CAD build for the part. Positions are in the model's coordinates, mm. Round coordinates to 2 decimals unless told otherwise and drop trailing zeros. Loops run counter-clockwise (first coordinate to the right, second up) from the corner with the lowest first, then second, coordinate; pieces in that order, holes last. Notation, with made-up numbers: (80.5, 83) - (120.5, 83) arc R14 ccw to (120.5, 96) - close; hole circle Ø6 at (-13, 14). An arc over 180 degrees is marked (long way). Use one line per item in the form item = value.
Autodesk Fusion 360 part; units mm, degrees
sketch "Sketch1" plane through (0, 0, 0) normal (0, 0, 1) x (1, 0, 0)
  circle A0 centre (0, 0) radius 7.5
  circle A1 centre (0, 0) radius 6.5
  dimension "d1" = 15
  dimension "d2" = -1
extrude "Extrude1" add sketch "Sketch1" along normal blind 497
equation "d3 = 527 mm - 30 mm"

Autodesk Fusion 360 part; units mm, degrees
sketch "Sketch1" plane through (0, 0, 0) normal (0, 0, 1) x (1, 0, 0)
  circle A0 centre (0, 0) radius 7.5
  circle A1 centre (0, 0) radius 6.5
  dimension "d1" = 15
  dimension "d2" = -1
extrude "Extrude1" add sketch "Sketch1" along normal blind 530
equation "d3 = 560 mm - 30 mm"

Autodesk Fusion 360 part; units mm, degrees
sketch "Sketch1" plane through (0, 0, 0) normal (0, 0, 1) x (1, 0, 0)
  line L0 (-29, 14) -> (29, 14)
  line L1 (29, 14) -> (29, -14)
  line L2 (29, -14) -> (-29, -14)
  line L3 (-29, -14) -> (-29, 14)
  line L4 (-29, 14) -> (29, -14) construction
  line L5 (29, 14) -> (-29, -14) construction
  dimension "d1" = 28
  dimension "d2" = 58
extrude "Extrude1" add sketch "Sketch1" along normal blind 175

Autodesk Fusion 360 part; units mm, degrees
sketch "Sketch1" plane through (0, 0, 0) normal (0, 0, 1) x (1, 0, 0)
  circle A0 centre (0, 0) radius 1.6
  line L0 (-3, -1.7321) -> (0, -3.4641)
  line L1 (0, -3.4641) -> (3, -1.7321)
  line L2 (3, -1.7321) -> (3, 1.7321)
  line L3 (3, 1.7321) -> (0, 3.4641)
  line L4 (0, 3.4641) -> (-3, 1.7321)
  line L5 (-3, 1.7321) -> (-3, -1.7321)
  dimension "d1" = 3.2
extrude "Extrude1" add sketch "Sketch1" along normal blind 25.3
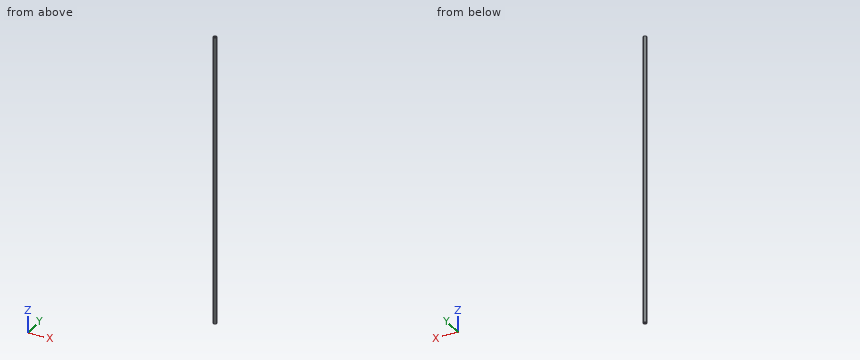
1) Slice it at A-A (y = 0). Write the cut outline in (x, z).
Report:
outline = (-3, 0) - (-1.6, 0) - (-1.6, 530) - (-3, 530) - close; (1.6, 0) - (3, 0) - (3, 530) - (1.6, 530) - close
2) Flat gauge pins, fed straight in: pin 1 (2 mm diameter, centred on y = 2, z = 243.5, fed in from +X); pin 2 (1 mm diameter, centred on x = -2, z = 91.5, fed in from -Y); pin 3 (3 mm diameter, centred on x = 1, z = 275, fed in from +Y). Where does each tip first touch, or does it go through?
Report:
pin_1 = 3
pin_2 = -2.6
pin_3 = 3.46
3) Drill centre lines: probe 1 along Y at (x, z) = (0, 279); probe 2 along Y at (x, z) = (0.9, 370); probe 3 along X at (y, z) = (0.75, 143). Where is each one in solid material? Low to high.
Report:
probe_1 = -3.46 to -1.6, 1.6 to 3.46
probe_2 = -2.94 to -1.32, 1.32 to 2.94
probe_3 = -3 to -1.41, 1.41 to 3
4) Slice it at B-B (z = 322). Write the cut outline in (x, y).
Report:
outline = (-3, -1.73) - (0, -3.46) - (3, -1.73) - (3, 1.73) - (0, 3.46) - (-3, 1.73) - close; hole circle Ø3.2 at (0, 0)
